```python
from build123d import *

# Parameters (mm, degrees)
EXTRUDE_1_DEPTH     = 12.2
CHAMFER_1_SIZE      = 1.5
CUT_EXTRUDE_1_DEPTH = 1.5
SKETCH_3_R          = 1.5
EXTRUDE_2_DEPTH     = 7
FILLET_1_R          = 2
SKETCH_4_R          = 3.5
EXTRUDE_3_DEPTH     = 7
EXTRUDE_3_TAPER     = 5
SKETCH_5_W          = 8
SKETCH_5_H          = 9
CUT_EXTRUDE_2_DEPTH = 2
SKETCH_6_R          = 2
SKETCH_6_W          = 6
SKETCH_6_H          = 1.5
CUT_EXTRUDE_3_DEPTH = 3


with BuildPart() as part:
    # 草图1 → 凸台-拉伸1 (new body)
    with BuildSketch(Plane(origin=(0, 0, 0), x_dir=(1, 0, 0), z_dir=(0, 1, 0))):
        Polygon((-32.25, 19), (-29.25, 22), (29.25, 22), (32.25, 19), (32.25, -19), (29.25, -22), (-29.25, -22), (-32.25, -19), align=None)
    extrude(amount=EXTRUDE_1_DEPTH)

    # 倒角1
    chamfer_1_edges = [part.edges().sort_by_distance(p)[0] for p in [
        (0, 12.2, 22),
        (30.75, 12.2, 20.5),
        (32.25, 12.2, 0),
        (30.75, 12.2, -20.5),
        (0, 12.2, -22),
        (-30.75, 12.2, -20.5),
        (-32.25, 12.2, 0),
        (-30.75, 12.2, 20.5),
    ]]
    chamfer(chamfer_1_edges, length=CHAMFER_1_SIZE)

    # 草图2 → 切除-拉伸1 (cut)
    with BuildSketch(Plane(origin=(0, 12.2, 0), x_dir=(1, 0, 0), z_dir=(0, 1, 0))):
        with BuildLine():
            Line((-25.75, 17.5), (25.75, 17.5))
            ThreePointArc((25.75, 17.5), (27.164213562, 16.914213562), (27.75, 15.5))
            Line((27.75, 15.5), (27.75, -15.5))
            ThreePointArc((27.75, -15.5), (27.164213562, -16.914213562), (25.75, -17.5))
            Line((25.75, -17.5), (-25.75, -17.5))
            ThreePointArc((-25.75, -17.5), (-27.164213562, -16.914213562), (-27.75, -15.5))
            Line((-27.75, -15.5), (-27.75, 15.5))
            ThreePointArc((-27.75, 15.5), (-27.164213562, 16.914213562), (-25.75, 17.5))
        make_face()
    extrude(amount=-CUT_EXTRUDE_1_DEPTH, mode=Mode.SUBTRACT)

    # 草图3 → 凸台-拉伸2 (add)
    # profile 1 of 2: a face of its own
    with BuildSketch(Plane.XZ):
        with BuildLine():
            Line((32.25, 9.5), (36.75, 9.5))
            ThreePointArc((36.75, 9.5), (37.810660172, 9.060660172), (38.25, 8))
            Line((38.25, 8), (38.25, 5))
            ThreePointArc((38.25, 5), (37.810660172, 3.939339828), (36.75, 3.5))
            Line((36.75, 3.5), (32.25, 3.5))
            Line((32.25, 3.5), (32.25, 9.5))
        make_face()
        with Locations(Location((35.25, 6.5, 0), (0, 0, 270))):
            Circle(SKETCH_3_R, mode=Mode.SUBTRACT)
    # profile 2 of 2: a face of its own
    with BuildSketch(Plane.XZ):
        with BuildLine():
            Line((-32.25, -3.5), (-36.75, -3.5))
            ThreePointArc((-36.75, -3.5), (-37.810660172, -3.939339828), (-38.25, -5))
            Line((-38.25, -5), (-38.25, -8))
            ThreePointArc((-38.25, -8), (-37.810660172, -9.060660172), (-36.75, -9.5))
            Line((-36.75, -9.5), (-32.25, -9.5))
            Line((-32.25, -9.5), (-32.25, -3.5))
        make_face()
        with Locations(Location((-35.25, -6.5, 0), (0, 0, 270))):
            Circle(SKETCH_3_R, mode=Mode.SUBTRACT)
    extrude(amount=-EXTRUDE_2_DEPTH)

    # 圆角1
    fillet_1_edges = [part.edges().sort_by_distance(p)[0] for p in [
        (32.25, 3.5, 3.5),
        (32.25, 3.5, 9.5),
        (-32.25, 3.5, -3.5),
        (-32.25, 3.5, -9.5),
    ]]
    fillet(fillet_1_edges, radius=FILLET_1_R)

    # 草图4 → 凸台-拉伸3 (add)
    with BuildSketch(Plane.XY.offset(22)):
        with Locations((9.75, 5)):
            Circle(SKETCH_4_R)
    extrude(amount=EXTRUDE_3_DEPTH, taper=EXTRUDE_3_TAPER)

    # 草图5 → 切除-拉伸2 (cut)
    with BuildSketch(Plane(origin=(0, 0, -22), x_dir=(-1, 0, 0), z_dir=(0, 0, -1))):
        with BuildLine():
            Line((-23.25, 4), (-23.25, 0))
            Line((-23.25, 0), (2.75, 0))
            Line((2.75, 0), (2.75, 4))
            ThreePointArc((2.75, 4), (-1.25, 8), (-5.25, 4))
            Line((-5.25, 4), (-6.25, 4))
            ThreePointArc((-6.25, 4), (-10.25, 8), (-14.25, 4))
            Line((-14.25, 4), (-15.25, 4))
            ThreePointArc((-15.25, 4), (-19.25, 8), (-23.25, 4))
        make_face()
        with Locations((13.25, 4.5)):
            Rectangle(SKETCH_5_W, SKETCH_5_H)
    extrude(amount=-CUT_EXTRUDE_2_DEPTH, mode=Mode.SUBTRACT)

    # 草图6 → 切除-拉伸3 (cut)
    with BuildSketch(Plane(origin=(0, 0, -20), x_dir=(-1, 0, 0), z_dir=(0, 0, -1))):
        with Locations((-19.25, 4)):
            Circle(SKETCH_6_R)
        with Locations((-10.25, 4)):
            Circle(SKETCH_6_R)
        with Locations((-1.25, 4)):
            Circle(SKETCH_6_R)
        with Locations((13.25, 7.25)):
            Rectangle(SKETCH_6_W, SKETCH_6_H)
    extrude(amount=-CUT_EXTRUDE_3_DEPTH, mode=Mode.SUBTRACT)


solid = part.part
```
Input: part model. Units: mm. Frame: model coordinates. A direction names the side the tool comes from. Coordinates: 2 decimals unless noted, no trailing zeros. Loops run counter-clockwise (first coordinate to the right, second up) from the corner with the lowest first, then second, coordinate; pieces in that order, holes last.
Q1. Section B-B, the plane z = 6.5. Return the cut outline in (x, y), and give its area (3 significant figures).
Results are:
outline: (-32.25, 0) - (33.75, 0) - (33.75, 7) - (32.25, 7) - (32.25, 10.7) - (30.75, 12.2) - (27.75, 12.2) - (27.75, 10.7) - (-27.75, 10.7) - (-27.75, 12.2) - (-30.75, 12.2) - (-32.25, 10.7) - close; (36.75, 0) - (38.25, 0) - (38.25, 7) - (36.75, 7) - close
area: 722 mm2
Q2. Set-up query: faces 4 (the flat face through (36, 3, 3.5)), 5 (the cylindrical face through (-37.8, 3.45, -3.93)), 6 (the flat face through (-9.25, 4, -21)), 7 (the flat face through (-13, 8, -19)), 8 (the flat face through (0, 11, 17.5)). Return all of +Z, -Z, +X, -X, +Y, -Y with unobstructed straight access to the full face (end or side cutting, diameter ignored); none if empty.
Results are:
face 4: -Z, +X, +Y, -Y
face 5: +Z, -X, +Y, -Y
face 6: -Z, -Y
face 7: -Z
face 8: +Y
Q3. Section C-C, the plane x = -11. Return the cut outline in (y, z), and give its area (3 significant figures).
Results are:
outline: (0, -20) - (6.5, -20) - (6.5, -17) - (8, -17) - (8, -20) - (9, -20) - (9, -22) - (10.7, -22) - (12.2, -20.5) - (12.2, -17.5) - (10.7, -17.5) - (10.7, 17.5) - (12.2, 17.5) - (12.2, 20.5) - (10.7, 22) - (0, 22) - close
area: 460 mm2
Q4. Section D-D, the plane x = -27. Return the cut outline in (y, z), and give its area (3 significant figures).
Results are:
outline: (0, -22) - (10.7, -22) - (12.2, -20.5) - (12.2, -17.06) - (10.7, -17.06) - (10.7, 17.06) - (12.2, 17.06) - (12.2, 20.5) - (10.7, 22) - (0, 22) - close
area: 483 mm2
Q5. Mould query, pull axis X, two halves, no side actions, for faces 1 (the flat face through (-38.25, 3, -6)), 2 (the flat face through (-10.25, 7, -19)), 3 (the flat face through (-36, 3, -9.5)). Classes: +X half, -X half, draft (parallel to the pull), parting line (faces both ways), or undercut.
Results are:
face 1: -X half
face 2: undercut
face 3: draft
Q6. Section A-A, the plane x = 35.25. Return the cut outline in (y, z).
Results are:
outline: (0, 3.5) - (7, 3.5) - (7, 5) - (0, 5) - close; (0, 8) - (7, 8) - (7, 9.5) - (0, 9.5) - close
Q7. Contact query for flat-ended pins moving along their axis: pin 1 (1 mm diameter, centred on y = 6.5, z = 6, fed in from -X); pin 2 (1.6 mm diameter, centred on y = 2.5, z = -21, fed in from -X); pin 3 (2 mm diameter, centred on x = 9.5, y = 4, fed in from -Z); pin 4 (2.5 mm diameter, centred on x = 35.25, z = 6.5, fed in from -Y). Output: stop coordinate, or through.
Results are:
pin 1: stops at x = -32.25
pin 2: stops at x = -31.05
pin 3: stops at z = -17
pin 4: passes through
Q8. Line query: line 1 along Y through (x, z) = (10, -19); line 2 along X through (y, z) = (4.5, 6.5); line 3 along X through (y, z) = (3.75, -6.5). Output: solid intervals per line, ascending.
Results are:
line 1: y = 0 to 2.02, 5.98 to 12.2
line 2: x = -32.25 to 33.75, 36.75 to 38.25
line 3: x = -38.25 to -36.75, -33.75 to 32.25
